Autodesk Inventor part; units mm, degrees
ref_plane "YZ Plane" through (0, 0, 0) normal (1, 0, 0) x (0, 1, 0)
ref_plane "XZ Plane" through (0, 0, 0) normal (0, 1, 0) x (-1, 0, 0)
ref_plane "XY Plane" through (0, 0, 0) normal (0, 0, 1) x (1, 0, 0)
sketch "Sketch1" plane through (0, 0, 0) normal (0, 1, 0) x (-1, 0, 0)
  line L0 (0, 0) -> (31.75, 0)
  line L1 (31.75, 0) -> (31.75, -38.1)
  line L2 (31.75, -38.1) -> (0, -38.1)
  line L3 (0, -38.1) -> (0, 0)
  dimension "d0" = 38.1
  dimension "d1" = 31.75
extrude "Extrusion1" add sketch "Sketch1" along normal blind 1.27
sketch "Sketch2" plane through (0, 1.27, 0) normal (0, 1, 0) x (1, 0, 0)
  circle A0 centre (-27.94, 3.81) radius 2.2225
  line L0 (-31.75, 38.1) -> (-31.75, 0)
  line L1 (-31.75, 19.05) -> (0, 19.05) construction
  line L2 (-31.75, 0) -> (0, 0)
  line L3 (-15.875, 0) -> (-15.875, 38.1) construction
  line L4 (0, 38.1) -> (-31.75, 38.1)
  circle A1 centre (-27.94, 34.29) radius 2.2225
  circle A2 centre (-3.81, 3.81) radius 2.2225
  circle A3 centre (-3.81, 34.29) radius 2.2225
  point P0 (-15.875, 19.05)
  dimension "d4" = 3.81
  dimension "d5" = 3.81
  dimension "d6" = 4.445
extrude "Extrusion2" cut sketch "Sketch2" against normal blind 1.27
sketch "Sketch3" plane through (0, 0, 0) normal (0, -1, 0) x (1, 0, 0)
  line L0 (-15.875, -25.4) -> (-15.875, -12.7)
  line L1 (-31.75, -38.1) -> (0, -38.1)
  line L2 (0, -38.1) -> (0, 0)
  line L3 (-15.875, -12.7) -> (-47.625, -12.7)
  line L4 (-47.625, -12.7) -> (-47.625, -25.4)
  line L5 (-47.625, -25.4) -> (-15.875, -25.4)
  line L6 (-15.875, -25.4) -> (-15.875, -12.7)
  dimension "d9" = 12.7
  dimension "d14" = 15.875
  dimension "d15" = 31.75
extrude "Extrusion3" add sketch "Sketch3" along normal blind 33.02
properties part number "caster"
Can you work these out from the model? Positions are in its coordinate system, mm. A direction names the side the tool comes from. Coordinates: 2 decimals unless noted, no trailing zeros. Write each loop counter-clockwise with the first axis right and the second up, starting at its lowest first coordinate (ties: lowest second). Pieces come first, ordered by that corner, then holes.
Q1. Imagine slicing it at C-C, the plane x = -3.81. List the corners of the cut face in (y, z) for me.
Results found:
outline: (0, -38.1) - (1.27, -38.1) - (1.27, -36.51) - (0, -36.51) - close; (0, -32.07) - (1.27, -32.07) - (1.27, -6.03) - (0, -6.03) - close; (0, -1.59) - (1.27, -1.59) - (1.27, 0) - (0, 0) - close
Q2. Imagine slicing it at A-A, the plane x = -27.94. List the corners of the cut face in (y, z) for me.
Results found:
outline: (-33.02, -25.4) - (0, -25.4) - (0, -32.07) - (1.27, -32.07) - (1.27, -6.03) - (0, -6.03) - (0, -12.7) - (-33.02, -12.7) - close; (0, -38.1) - (1.27, -38.1) - (1.27, -36.51) - (0, -36.51) - close; (0, -1.59) - (1.27, -1.59) - (1.27, 0) - (0, 0) - close
Q3. Imagine slicing it at D-D, the plane z = -24.5. List the corners of the cut face in (x, y) for me (3 decimals).
Results found:
outline: (-47.625, -33.02) - (-15.875, -33.02) - (-15.875, 0) - (0, 0) - (0, 1.27) - (-31.75, 1.27) - (-31.75, 0) - (-47.625, 0) - close
Q4. If we mould it in two halves opening along Z, with no side actions, what happens to faces 1 (the face through (-47.625, -16, -19)), 2 (the face through (-2.78, 0.64, -1.84)), 3 (the face through (-28.229, 0.644, -36.494)), 4 (the face through (-32, -16, -12.7))? For each: +Z half, -Z half, draft (parallel to the pull), parting line (faces both ways), or undercut.
Results found:
face 1: draft
face 2: undercut
face 3: undercut
face 4: +Z half
Q5. For P1, Ø5, axis at x = -27.94, z = -34.29, coming from the -Y side; P2, Ø4, axis at x = -3.81, z = -34.29, coming from the +Y side; P3, Ø4, axis at y = -14.5, z = -21.5, coming from the +X side (3 decimals); P4, Ø2, axis at x = -23, y = -20, coming from the +Z side, each with a flat end and sliding along its axis, tell me the tip position at first contact or that it passes through.
Results found:
P1: stops at y = 0
P2: passes through
P3: stops at x = -15.875
P4: stops at z = -12.7
Q6. Which directions (+Z, -Z, +X, -X, +Y, -Y) give clear straight access to the entire face, cutting with the end or side of a thin tool? Please do faces 5 (the face through (-32, -16, -25.4)), 6 (the face through (-15.875, -16, -19)), 7 (the face through (0, 1, -19)), 8 (the face through (-31.75, 1, -19)).
Results found:
face 5: -Z, +X, -X, -Y
face 6: +Z, -Z, +X, -Y
face 7: +Z, -Z, +X, +Y, -Y
face 8: +Z, -Z, -X, +Y
Q7. Imagine slicing it at B-B, the plane z = -34.29. List the corners of the cut face in (x, y) for me, plus the area to 3 significant figures.
Results found:
outline: (-31.75, 0) - (-30.16, 0) - (-30.16, 1.27) - (-31.75, 1.27) - close; (-25.72, 0) - (-6.03, 0) - (-6.03, 1.27) - (-25.72, 1.27) - close; (-1.59, 0) - (0, 0) - (0, 1.27) - (-1.59, 1.27) - close
area: 29.0 mm2
Q8. Please list where these lines run through material, in increasing order: L1, parallel to Z at x = -27.94, y = 0.9; L2, parallel to X at y = 0.45, z = -34.29; L3, parallel to X at y = -17, z = -18.5 (3 decimals).
Results found:
L1: z = -38.1 to -36.51, -32.07 to -6.03, -1.59 to 0
L2: x = -31.75 to -30.16, -25.72 to -6.03, -1.59 to 0
L3: x = -47.625 to -15.875
